Could you check a few things on this model? Use its own coordinates, in mm. Face numbers are marked on the shaded views. A direction names the side the tool comes from. Round coordinates to 2 decimals unless told otherwise and drop trailing zeros. Loops run counter-clockwise (first coordinate to the right, second up) from the corner with the lowest first, then second, coordinate; pieces in that order, holes last. Notation, with made-up numbers: M 73,55 L 123,55 A7 cw 123,65 Z; hole C -21,38 d1. An arc over 180 degrees is marked long. One line per item, written item: value. Start each with the question number.
Q1. Imagine slicing it at B-B (x = -34.7). Please give me the cut outline in (y, z), then the cut area to 3 significant figures.
Q2. Thinking about a two-plate mould opening in Y: for the marked faces 1, 2 and 3, which applies, released by +Y, released by -Y, zero draft, split by the parting line, or undercut?
Q3. Which directions (+Z, -Z, +X, -X, +Y, -Y) give clear straight access to the entire face, cutting with the end or side of a thin tool? Please do the marked faces 4, 5 and 6.
Q4. Imagine slicing it at C-C (z = 7.75). Please give me the cut outline in (x, y), then the cut area to 3 significant figures.
Q5. Imagine slicing it at A-A (x = 13.8). Please give me the cut outline in (y, z).
Q6. Imagine slicing it at D-D (x = 0). Please give me the cut outline in (y, z).
Q7. Please list where these lines run through material, in increasing order: line 1 along Z through (x, y) = (-34.7, 27.95); line 2 along Z through (x, y) = (-34, 28); line 3 along Y through (x, z) = (10.5, -1.25).
Q8. I'm going to push flat-ended pins straight in: pin 1 Ø1 at (y, z) = (6, 8) entering from -X; pin 2 Ø1.5 at (y, z) = (5.5, 0) entering from +X; pin 3 Ø6 at (x, z) = (-8, 4.5) entering from +Y. Where does each tip first touch, or does it pass through?
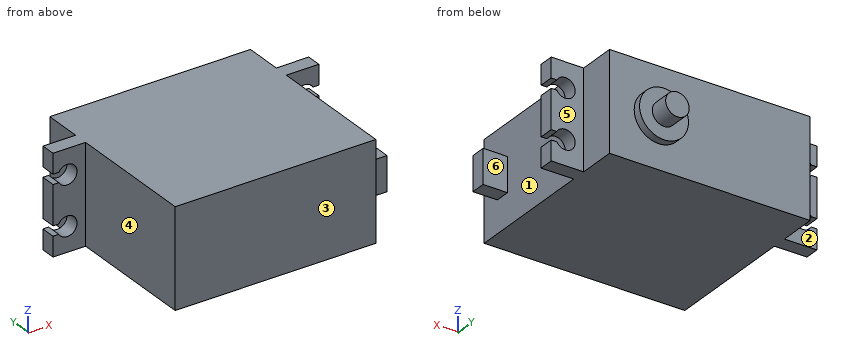
from build123d import *

# Parameters (mm, degrees)
BOSS_EXTRUDE1_START = -10.05
BOSS_EXTRUDE1_DEPTH = 20.1
CUT_EXTRUDE1_DEPTH  = 30.8
SKETCH5_R           = 5
BOSS_EXTRUDE2_DEPTH = 1.6
SKETCH6_R           = 2.4
BOSS_EXTRUDE3_DEPTH = 4
SKETCH8_W           = 7
SKETCH8_H           = 3
BOSS_EXTRUDE4_DEPTH = 5


with BuildPart() as part:
    # Sketch3 → Boss-Extrude1 (new body)
    with BuildSketch(Plane.XY.offset(BOSS_EXTRUDE1_START)):
        Polygon((-30.95, 0), (-30.95, 26.8), (-37.6, 26.8), (-37.6, 29.8), (-30.95, 29.8), (-30.95, 37.5), (10.05, 37.5), (10.05, 29.8), (16.7, 29.8), (16.7, 26.8), (10.05, 26.8), (10.05, 0), align=None)
    extrude(amount=BOSS_EXTRUDE1_DEPTH)

    # Sketch4 → Cut-Extrude1 (cut, through all)
    with BuildSketch(Plane(origin=(0, 29.8, 0), x_dir=(1, 0, 0), z_dir=(0, 1, 0))):
        with BuildLine():
            Line((-37.6, 6), (-37.6, 4))
            Line((-37.6, 4), (-36.432050808, 4))
            ThreePointArc((-36.432050808, 4), (-32.7, 5), (-36.432050808, 6))
            Line((-36.432050808, 6), (-37.6, 6))
        make_face()
        with BuildLine():
            Line((16.7, -6), (15.532050808, -6))
            ThreePointArc((15.532050808, -6), (11.8, -5), (15.532050808, -4))
            Line((15.532050808, -4), (16.7, -4))
            Line((16.7, -4), (16.7, -6))
        make_face()
        with BuildLine():
            Line((-37.6, -4), (-37.6, -6))
            Line((-37.6, -6), (-36.432050808, -6))
            ThreePointArc((-36.432050808, -6), (-32.7, -5), (-36.432050808, -4))
            Line((-36.432050808, -4), (-37.6, -4))
        make_face()
        with BuildLine():
            Line((16.7, 4), (15.532050808, 4))
            ThreePointArc((15.532050808, 4), (11.8, 5), (15.532050808, 6))
            Line((15.532050808, 6), (16.7, 6))
            Line((16.7, 6), (16.7, 4))
        make_face()
    extrude(amount=-CUT_EXTRUDE1_DEPTH, mode=Mode.SUBTRACT)

    # Sketch5 → Boss-Extrude2 (add)
    with BuildSketch(Plane(origin=(0, 37.5, 0), x_dir=(1, 0, 0), z_dir=(0, 1, 0))):
        Circle(SKETCH5_R)
    extrude(amount=BOSS_EXTRUDE2_DEPTH)

    # Sketch6 → Boss-Extrude3 (add)
    with BuildSketch(Plane(origin=(0, 39.1, 0), x_dir=(1, 0, 0), z_dir=(0, 1, 0))):
        Circle(SKETCH6_R)
    extrude(amount=BOSS_EXTRUDE3_DEPTH)

    # Sketch8 → Boss-Extrude4 (add)
    with BuildSketch(Plane(origin=(10.05, 0, 0), x_dir=(0, 0, -1), z_dir=(1, 0, 0))):
        with Locations((0, 5.5)):
            Rectangle(SKETCH8_W, SKETCH8_H)
    extrude(amount=BOSS_EXTRUDE4_DEPTH)


solid = part.part
Report:
1. outline: M 26.8,-10.05 L 29.8,-10.05 L 29.8,-7 L 26.8,-7 Z; M 26.8,-3 L 29.8,-3 L 29.8,3 L 26.8,3 Z; M 26.8,7 L 29.8,7 L 29.8,10.05 L 26.8,10.05 Z
1. area: 36.3 mm²
2. face 1: undercut
2. face 2: released by +Y
2. face 3: released by -Y
3. face 4: +Z, -Z, -X, -Y
3. face 5: +Z, -Z, +X, +Y
3. face 6: +Z, -Z, +X
4. outline: M -37.6,26.8 L -30.95,26.8 L -30.95,0 L 10.05,0 L 10.05,26.8 L 16.7,26.8 L 16.7,29.8 L 10.05,29.8 L 10.05,37.5 L -30.95,37.5 L -30.95,29.8 L -37.6,29.8 Z
4. area: 1,580 mm²
5. outline: M 4,-3.5 L 7,-3.5 L 7,3.5 L 4,3.5 Z; M 26.8,-10.05 L 29.8,-10.05 L 29.8,-7 L 26.8,-7 Z; M 26.8,-3 L 29.8,-3 L 29.8,3 L 26.8,3 Z; M 26.8,7 L 29.8,7 L 29.8,10.05 L 26.8,10.05 Z
6. outline: M 0,-10.05 L 37.5,-10.05 L 37.5,-5 L 39.1,-5 L 39.1,-2.4 L 43.1,-2.4 L 43.1,2.4 L 39.1,2.4 L 39.1,5 L 37.5,5 L 37.5,10.05 L 0,10.05 Z
7. line 1: z = -10.05 to -7, -3 to 3, 7 to 10.05
7. line 2: z = -10.05 to -6.87, -3.13 to 3.13, 6.87 to 10.05
7. line 3: y = 4 to 7, 26.8 to 29.8
8. pin 1: stops at x = -30.95
8. pin 2: stops at x = 15.05
8. pin 3: stops at y = 37.5
